Build history of the part. All positions in model axes, mm. Face numbers are marked on the shaded views. A direction names the side the tool comes from. Round coordinates to 2 decimals unless told otherwise and drop trailing zeros. Order: outer loops, then holes, each group sorted by start corner. A loop starts at its lowest first (then second) coordinate and runs counter-clockwise, first axis right, second up. Notation, with made-up numbers: (49.5, 85) -> (79.5, 85) arc R20 cw to (79.5, 91) -> close; hole circle Ø8 at (16.25, -32). An arc over 180 degrees is marked (long way). Answer as a JSON object with one key per item and string values.
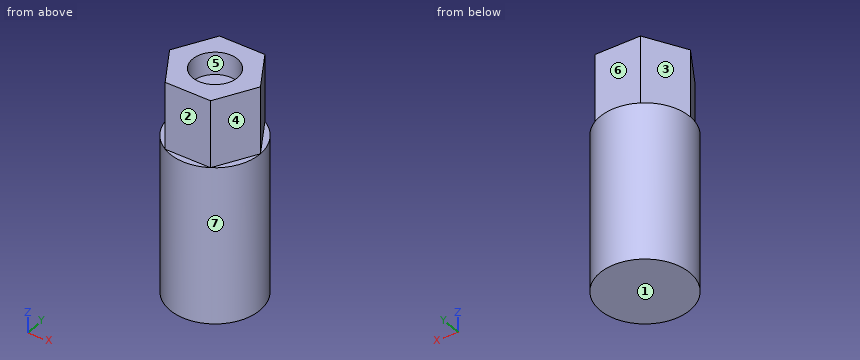
from build123d import *

# Parameters (mm, degrees)
F0_R     = 25.4
F1_DEPTH = 127
F3_DEPTH = 38.1
F4_R     = 12.7
F5_DEPTH = 12.7


with BuildPart() as f1:
    # F0 (on Top) → F1 (new body)
    with BuildSketch(Plane.XY):
        Circle(F0_R)
    extrude(amount=F1_DEPTH)

    # F2 (on face) → F3 (cut)
    with BuildSketch(Plane.XY.offset(127)):
        with BuildLine():
            ThreePointArc((-25.4, 0), (-21.997045, -12.7), (-12.7, -21.997045))
            Line((-12.7, -21.997045), (-25.4, 0))
        make_face()
        with BuildLine():
            ThreePointArc((-12.7, -21.997045), (0, -25.4), (12.7, -21.997045))
            Line((12.7, -21.997045), (-12.7, -21.997045))
        make_face()
        with BuildLine():
            ThreePointArc((12.7, -21.997045), (21.997045, -12.7), (25.4, 0))
            Line((25.4, 0), (12.7, -21.997045))
        make_face()
        with BuildLine():
            Line((12.7, 21.997045), (25.4, 0))
            ThreePointArc((25.4, 0), (21.997045, 12.7), (12.7, 21.997045))
        make_face()
        with BuildLine():
            Line((-12.7, 21.997045), (12.7, 21.997045))
            ThreePointArc((12.7, 21.997045), (0, 25.4), (-12.7, 21.997045))
        make_face()
        with BuildLine():
            Line((-25.4, 0), (-12.7, 21.997045))
            ThreePointArc((-12.7, 21.997045), (-21.997045, 12.7), (-25.4, 0))
        make_face()
    extrude(amount=-F3_DEPTH, mode=Mode.SUBTRACT)

    # F4 (on face) → F5 (cut, symmetric)
    with BuildSketch(Plane.XY.offset(127)):
        Circle(F4_R)
    extrude(amount=F5_DEPTH, both=True, mode=Mode.SUBTRACT)


solid = f1.part
1) Flat gauge pins, fed straight in: pin 1 Ø4 at (x, y) = (20.5, 13.5) entering from +Z; pin 2 Ø1 at (y, z) = (-9.5, 99) entering from -X; pin 3 Ø12 at (y, z) = (-7, 41) entering from +X. Where does each tip first touch, or does it go through?
Checked values:
{"pin 1": "stops at z = 88.9", "pin 2": "stops at x = -20.2", "pin 3": "stops at x = 25.38"}
2) Cut at B-B, the plane y = -9. Give the cut face in (x, z), plus the area to 3 significant figures.
Checked values:
{"outline": "(-23.75, 0) -> (23.75, 0) -> (23.75, 88.9) -> (20.2, 88.9) -> (20.2, 127) -> (8.96, 127) -> (8.96, 114.3) -> (-8.96, 114.3) -> (-8.96, 127) -> (-20.2, 127) -> (-20.2, 88.9) -> (-23.75, 88.9) -> close", "area": "5,540 mm²"}
3) Probe L1, parallel to Y at x = 0, z = 117; L2, parallel to Z at x = -11, y = 4.5; L3, parallel to Z at x = 20, y = -15. List the from-to ranges inside material, lowest first. Write a range as from..to.
Checked values:
{"L1": "y = -22..-12.7, 12.7..22", "L2": "z = 0..114.3", "L3": "z = 0..88.9"}
4) Cut at C-C, the plane z = 71. Give the cut face in (x, y), plus the area to 3 significant figures.
Checked values:
{"outline": "circle Ø50.8 at (0, 0)", "area": "2,030 mm²"}
5) Which spindle directions (+Z, -Z, +X, -X, +Y, -Y) get a long thin tool onto all of the face, cutting with end or side? Do the marked faces 1, 2 and 3. Say none if no direction does.
Checked values:
{"face 1": "-Z, +X, -X, +Y, -Y", "face 2": "+Z, +X, -X, -Y", "face 3": "+Z, -X, +Y"}
6) Cut at A-A, the plane x = 0. Give the cut face in (y, z).
Checked values:
{"outline": "(-25.4, 0) -> (25.4, 0) -> (25.4, 88.9) -> (22, 88.9) -> (22, 127) -> (12.7, 127) -> (12.7, 114.3) -> (-12.7, 114.3) -> (-12.7, 127) -> (-22, 127) -> (-22, 88.9) -> (-25.4, 88.9) -> close"}
7) Pull direction X, two halves, no side cores. Call the marked faces 4, 5, 6 and 7: pulls with the +X half, pulls with the -X half, needs draft (parallel to the pull), parting line crosses it, or undercut.
Checked values:
{"face 4": "pulls with the +X half", "face 5": "undercut", "face 6": "needs draft", "face 7": "parting line crosses it"}
8) Cut at D-D, the plane y = -16. Give the cut face in (x, z), plus the area to 3 significant figures.
Checked values:
{"outline": "(-19.73, 0) -> (19.73, 0) -> (19.73, 88.9) -> (16.16, 88.9) -> (16.16, 127) -> (-16.16, 127) -> (-16.16, 88.9) -> (-19.73, 88.9) -> close", "area": "4,740 mm²"}
